Build history of the part. All positions in model axes, mm. A direction names the side the tool comes from. Round coordinates to 2 decimals unless told otherwise and drop trailing zeros. Order: outer loops, then holes, each group sorted by start corner. A loop starts at its lowest first (then second) coordinate and runs counter-clockwise, first axis right, second up. Notation, with made-up numbers: (82.25, 73) -> (140.25, 73) arc R20 ccw to (140.25, 103) -> close; hole circle Ø5 at (83.5, 62). An arc over 180 degrees is marked (long way). Answer as a JSON object with one key per item and string values.
from build123d import *

# Parameters (mm, degrees)
F0_R     = 34.032564
F1_DEPTH = 25
F3_DEPTH = 25


with BuildPart() as f1:
    # F0 (on Top) → F1 (new body)
    with BuildSketch(Plane.XY):
        with Locations((3.729817, 0)):
            Circle(F0_R)
    extrude(amount=F1_DEPTH)

    # F2 (on face) → F3 (join)
    with BuildSketch(Plane.XY.offset(25)):
        Polygon((2.597546, 49.992847), (-12.253506, 48.537445), (-26.015781, 42.769278), (-37.466439, 33.200873), (-45.588039, 20.682425), (-49.658942, 6.326253), (-49.31743, -8.592035), (-44.593849, -22.746883), (-35.907907, -34.880571), (-24.031391, -43.914966), (-10.01958, -49.047324), (4.882514, -49.821613), (19.350776, -46.169032), (32.099636, -38.41413), (41.996303, -27.245964), (48.161414, -13.656875), (50.047172, 1.145688), (47.486019, 15.846451), (40.705525, 29.139187), (30.308167, 39.842779), (17.217794, 47.006165), align=None)
    extrude(amount=F3_DEPTH)


solid = f1.part
1) Cut at B-B, the plane y = -19. Give the cut face in (x, z).
Checked values:
{"outline": "(-45.84, 25) -> (-24.51, 25) -> (-24.51, 0) -> (31.96, 0) -> (31.96, 25) -> (45.74, 25) -> (45.74, 50) -> (-45.84, 50) -> close"}
2) Probe L1, parallel to Z at x = 6.5, y = -34; L2, parallel to Y at x = 2.5, z = 16; L3, parallel to X at y = 29, z = 21.5. List the from-to ranges inside material, lowest first. Write a range as from..to.
Checked values:
{"L1": "z = 25..50", "L2": "y = -34.01..34.01", "L3": "x = -14.08..21.54"}
3) Cut at A-A, the plane z = 31.5. Give the cut face in (x, y).
Checked values:
{"outline": "(-49.66, 6.33) -> (-49.32, -8.59) -> (-44.59, -22.75) -> (-35.91, -34.88) -> (-24.03, -43.91) -> (-10.02, -49.05) -> (4.88, -49.82) -> (19.35, -46.17) -> (32.1, -38.41) -> (42, -27.25) -> (48.16, -13.66) -> (50.05, 1.15) -> (47.49, 15.85) -> (40.71, 29.14) -> (30.31, 39.84) -> (17.22, 47.01) -> (2.6, 49.99) -> (-12.25, 48.54) -> (-26.02, 42.77) -> (-37.47, 33.2) -> (-45.59, 20.68) -> close"}
4) Flat gauge pins, fed straight in: pin 1 Ø1 at (y, z) = (-20, 8.5) entering from -X; pin 2 Ø3 at (x, z) = (6, 5) entering from +Y; pin 3 Ø6 at (y, z) = (-10, 11.5) entering from +X; pin 4 Ø12 at (y, z) = (4.5, 34.5) entering from +X. Where does each tip first touch, or does it go through?
Checked values:
{"pin 1": "stops at x = -24.16", "pin 2": "stops at y = 34.02", "pin 3": "stops at x = 37.03", "pin 4": "stops at x = 50.05"}
5) Which spindle directions (+Z, -Z, +X, -X, +Y, -Y) get a long thin tool onto all of the face, cutting with end or side? Do faces 1 (the face through (-41.47, 27.03, 37.33)), 2 (the face through (-23, 23, 25)). Say none if no direction does.
Checked values:
{"face 1": "+Z, -Z, -X, +Y", "face 2": "-Z"}
6) Cut at C-C, the plane x = -21. Give the cut face in (y, z).
Checked values:
{"outline": "(-45.03, 25) -> (-23.38, 25) -> (-23.38, 0) -> (23.38, 0) -> (23.38, 25) -> (44.87, 25) -> (44.87, 50) -> (-45.03, 50) -> close"}
7) Cut at D-D, the plane z = 15. Give the cut face in (x, y).
Checked values:
{"outline": "circle Ø68.07 at (3.73, 0)"}
